```python
from build123d import *

# Parameters (mm, degrees)
ESBO_O1_R                = 28.575
ESBO_O1_R_2              = 26.575
RESSALTO_EXTRUS_O1_DEPTH = 32
ESBO_O2_R                = 4
CORTE_EXTRUS_O1_DEPTH    = 32
PADR_OCIRCULAR1_COUNT    = 6


with BuildPart() as part:
    # Esboço1 → Ressalto-extrusão1 (new body)
    with BuildSketch(Plane.XY):
        Circle(ESBO_O1_R)
        Circle(ESBO_O1_R_2, mode=Mode.SUBTRACT)
    extrude(amount=RESSALTO_EXTRUS_O1_DEPTH)

    # Esboço2 → Corte-extrusão1 (cut)
    with BuildSketch(Plane(origin=(0, 0, 0), x_dir=(0, 0, -1), z_dir=(1, 0, 0))):
        with Locations((-16, 0)):
            Circle(ESBO_O2_R)
    corte_extrus_o1 = extrude(amount=-CORTE_EXTRUS_O1_DEPTH, mode=Mode.SUBTRACT)

    # PadrãoCircular1: Corte-extrusão1 ×6 about axis
    padr_ocircular1_axis = Axis((0, 0, 32), (0, 0, -1))
    for i in range(1, PADR_OCIRCULAR1_COUNT):
        add(corte_extrus_o1.rotate(padr_ocircular1_axis, i * 360 / PADR_OCIRCULAR1_COUNT), mode=Mode.SUBTRACT)


solid = part.part
```
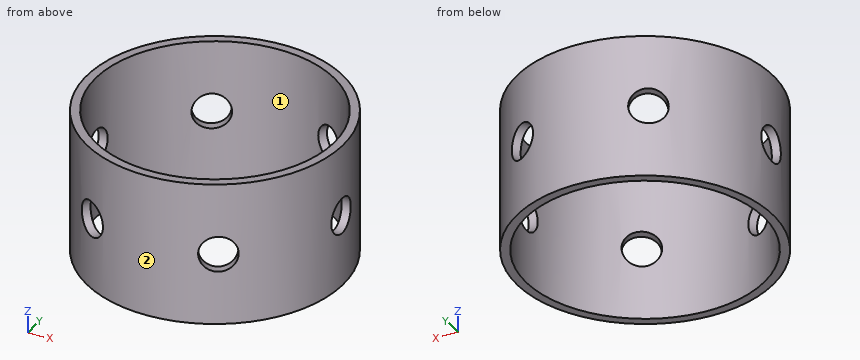
Geometry check sheet. Reference: the model listing, model coordinates, mm. Face numbers are marked on the shaded views. Coordinates: 2 decimals unless noted, no trailing zeros. Loops run counter-clockwise (first coordinate to the right, second up) from the corner with the lowest first, then second, coordinate; pieces in that order, holes last.
Item 1: Thickness scan on line 1 (Y direction, x = 0, z = 23.5) (3 decimals); line 2 (Y direction, x = 7, z = 23); line 3 (X direction, y = 15.5, z = 29). Record the ranges inside material, lowest first.
Item 2: Release check for a two-part mould opening along X. For the marked faces 1 and 2 record: released by +X, released by -X, zero draft, split by the parting line, or undercut.
Item 3: Sectioned sample at C-C, the plane z = 15.5. Record the boundary of the cut face in (x, y) (3 decimals).
Item 4: Go/stop test with flat-tipped pins: pin 1 Ø10 at (x, z) = (-22.5, 13) entering from -Y; pin 2 Ø4 at (y, z) = (-8.5, 16.5) entering from -X; pin 3 Ø2 at (y, z) = (15, 24) entering from +X; pin 4 Ø6.5 at (y, z) = (0, 16) entering from -X. Record where each tip stops, or that it passes through.
Item 5: Sectioned sample at D-D, the plane y = -13. Record the boundary of the cut face in (x, z).
Item 6: Sectioned sample at B-B, the plane x = 0. Record the boundary of the cut face in (y, z) (3 decimals), then the cut area to 3 significant figures.
Item 7: Sectioned sample at A-A, the plane y = 0. Record the boundary of the cut face in (x, z) (3 decimals), then the cut area to 3 significant figures.
Check result:
1. line 1: y = -28.575 to -26.575, 26.575 to 28.575
1. line 2: y = -27.7 to -25.64, 25.64 to 27.7
1. line 3: x = -24.01 to -21.59, 21.59 to 24.01
2. face 1: undercut
2. face 2: split by the parting line
3. outline: (-28.298, -3.969) arc R28.575 ccw to (-17.586, -22.523) - (-16.575, -20.772) arc R26.575 cw to (-26.277, -3.969) - close; (-28.298, 3.969) - (-26.277, 3.969) arc R26.575 cw to (-16.575, 20.772) - (-17.586, 22.523) arc R28.575 ccw to start; (-10.712, -26.491) arc R28.575 ccw to (10.712, -26.491) - (9.702, -24.741) arc R26.575 cw to (-9.702, -24.741) - close; (-10.712, 26.491) - (-9.702, 24.741) arc R26.575 cw to (9.702, 24.741) - (10.712, 26.491) arc R28.575 ccw to start; (16.575, -20.772) - (17.586, -22.523) arc R28.575 ccw to (28.298, -3.969) - (26.277, -3.969) arc R26.575 cw to start; (16.575, 20.772) arc R26.575 cw to (26.277, 3.969) - (28.298, 3.969) arc R28.575 ccw to (17.586, 22.523) - close
4. pin 1: stops at y = -22.59
4. pin 2: stops at x = -27.83
4. pin 3: stops at x = 24.91
4. pin 4: passes through
5. outline: (-25.45, 0) - (-23.18, 0) - (-23.18, 32) - (-25.45, 32) - close; (23.18, 0) - (25.45, 0) - (25.45, 32) - (23.18, 32) - close
6. outline: (-28.575, 0) - (-26.575, 0) - (-26.575, 32) - (-28.575, 32) - close; (26.575, 0) - (28.575, 0) - (28.575, 32) - (26.575, 32) - close
6. area: 128 mm2
7. outline: (-28.575, 0) - (-26.575, 0) - (-26.575, 12) - (-28.575, 12) - close; (-28.575, 20) - (-26.575, 20) - (-26.575, 32) - (-28.575, 32) - close; (26.575, 0) - (28.575, 0) - (28.575, 12) - (26.575, 12) - close; (26.575, 20) - (28.575, 20) - (28.575, 32) - (26.575, 32) - close
7. area: 96.0 mm2
